For this review, take the finished solid that the model builds, in its own axes (mm). Face numbers are marked on the shaded views. A direction names the side the tool comes from. Coordinates: 2 decimals unless noted, no trailing zeros. Order: outer loops, then holes, each group sorted by start corner. A loop starts at its lowest first (then second) coordinate and runs counter-clockwise, first axis right, second up. Notation, with made-up numbers: (-39, 62.5) -> (13, 62.5) arc R11 cw to (13, 75.5) -> close; hole circle Ø10 at (70, 45.25). An arc over 180 degrees is marked (long way). Answer as a JSON object with one key per item and string values. Group by question number.
1) Draft analysis for pull direction X (two halves, no side actions). For the marked faces 1, 2, 3 and 4, state which applies: +X half, -X half, draft (parallel to the pull), parting line (faces both ways), or undercut.
2) Add section B-B, the plane y = -16. Count the separate pieces of the cut face and the enclosed holes in it, then the cut area to 3 significant figures.
3) Add section A-A, the plane z = 1.25. Write out the cut boundary in (x, y), then the cut area to 3 significant figures.
4) Machinability: for the marked faces 5 and 6, which of the approach directions +Z, -Z, +X, -X, +Y, -Y give a long, thin tool a straight path to every point of the face, cutting with its end or side? Answer none if there is none.
5) Wall thickness on L1, parallel to X at y = 12.5, z = 1; L2, parallel to Y at x = -24.5, z = 2; L3, parallel to Z at x = 32, y = -12.5: over which ranges is each line inside the solid? List them lowest first.
6) For pin 1 (6.5 mm diameter, centred on x = 0, y = 24, fed in from -Z); pin 2 (11 mm diameter, centred on x = 0, y = -8, fed in from +Z), all flat-tipped, find the tip position at first contact; note any pin that passes through.
from build123d import *

# Parameters (mm, degrees)
EXTRUDE_THIN1_DEPTH       = 10
BOSS_EXTRUDE1_DEPTH       = 2
SKETCH3_W                 = 3
SKETCH3_H                 = 56
BOSS_EXTRUDE2_DEPTH       = 6.5
SKETCH4_W                 = 9
SKETCH4_H                 = 56
BOSS_EXTRUDE3_DEPTH       = 5
F_3_0MM_DOWEL_HOLE1_D     = 3
F_3_0MM_DOWEL_HOLE1_DEPTH = 150
SKETCH10_R                = 3.5
CUT_EXTRUDE1_DEPTH        = 65.195015383
CUT_EXTRUDE1_DEPTH_BACK   = 65.195015383
BOSS_EXTRUDE4_REACH       = 105.179
SKETCH12_W                = 9
SKETCH12_H                = 56
SKETCH12_R                = 1.5
BOSS_EXTRUDE5_REACH       = 105.179
SKETCH13_W                = 9
SKETCH13_H                = 56
SKETCH13_R                = 1.5
SKETCH14_R                = 1.5
CUT_EXTRUDE2_DEPTH        = 104.179455319
CUT_EXTRUDE2_DEPTH_BACK   = 104.179455319
SKETCH15_R                = 1.5
SKETCH15_R_2              = 1.2
BOSS_EXTRUDE6_DEPTH       = 8.5
BOSS_EXTRUDE7_START       = -100
SKETCH15_2_R              = 1.5
SKETCH15_2_R_2            = 1.2
BOSS_EXTRUDE7_DEPTH       = 8.5


with BuildPart() as part:
    # Sketch1 → Extrude-Thin1 (new body)
    with BuildSketch(Plane.XY):
        with BuildLine():
            Line((-35.5, 39), (35.5, 39))
            ThreePointArc((35.5, 39), (41.156854249, 36.656854249), (43.5, 31))
            Line((43.5, 31), (43.5, -31))
            ThreePointArc((43.5, -31), (41.156854249, -36.656854249), (35.5, -39))
            Line((35.5, -39), (-35.5, -39))
            ThreePointArc((-35.5, -39), (-41.156854249, -36.656854249), (-43.5, -31))
            Line((-43.5, -31), (-43.5, 31))
            ThreePointArc((-43.5, 31), (-41.156854249, 36.656854249), (-35.5, 39))
        make_face()
        with BuildLine():
            Line((-35.5, 37), (35.5, 37))
            ThreePointArc((35.5, 37), (39.742640687, 35.242640687), (41.5, 31))
            Line((41.5, 31), (41.5, -31))
            ThreePointArc((41.5, -31), (39.742640687, -35.242640687), (35.5, -37))
            Line((35.5, -37), (-35.5, -37))
            ThreePointArc((-35.5, -37), (-39.742640687, -35.242640687), (-41.5, -31))
            Line((-41.5, -31), (-41.5, 31))
            ThreePointArc((-41.5, 31), (-39.742640687, 35.242640687), (-35.5, 37))
        make_face(mode=Mode.SUBTRACT)
    extrude(amount=EXTRUDE_THIN1_DEPTH)

    # Sketch2 → Boss-Extrude1 (add)
    with BuildSketch(Plane(origin=(0, 0, 0), x_dir=(-1, 0, 0), z_dir=(0, 0, -1))):
        with BuildLine():
            Line((35.5, 39), (-35.5, 39))
            ThreePointArc((-35.5, 39), (-41.156854249, 36.656854249), (-43.5, 31))
            Line((-43.5, 31), (-43.5, -31))
            ThreePointArc((-43.5, -31), (-41.156854249, -36.656854249), (-35.5, -39))
            Line((-35.5, -39), (35.5, -39))
            ThreePointArc((35.5, -39), (41.156854249, -36.656854249), (43.5, -31))
            Line((43.5, -31), (43.5, 31))
            ThreePointArc((43.5, 31), (41.156854249, 36.656854249), (35.5, 39))
        make_face()
        with BuildLine():
            ThreePointArc((-35.5, -37), (-39.742640687, -35.242640687), (-41.5, -31))
            Line((-41.5, -31), (-41.5, 31))
            ThreePointArc((-41.5, 31), (-39.742640687, 35.242640687), (-35.5, 37))
            Line((-35.5, 37), (35.5, 37))
            ThreePointArc((35.5, 37), (39.742640687, 35.242640687), (41.5, 31))
            Line((41.5, 31), (41.5, -31))
            ThreePointArc((41.5, -31), (39.742640687, -35.242640687), (35.5, -37))
            Line((35.5, -37), (-35.5, -37))
        make_face(mode=Mode.SUBTRACT)
        with BuildLine():
            Line((-41.5, -31), (-41.5, 31))
            ThreePointArc((-41.5, 31), (-39.742640687, 35.242640687), (-35.5, 37))
            Line((-35.5, 37), (35.5, 37))
            ThreePointArc((35.5, 37), (39.742640687, 35.242640687), (41.5, 31))
            Line((41.5, 31), (41.5, -31))
            ThreePointArc((41.5, -31), (39.742640687, -35.242640687), (35.5, -37))
            Line((35.5, -37), (-35.5, -37))
            ThreePointArc((-35.5, -37), (-39.742640687, -35.242640687), (-41.5, -31))
        make_face()
    extrude(amount=BOSS_EXTRUDE1_DEPTH)

    # Sketch3 → Boss-Extrude2 (add)
    with BuildSketch(Plane.ZY.offset(43.5)):
        with Locations((-0.5, 0)):
            Rectangle(SKETCH3_W, SKETCH3_H)
    boss_extrude2 = extrude(amount=BOSS_EXTRUDE2_DEPTH)

    # Sketch4 → Boss-Extrude3 (add)
    with BuildSketch(Plane.ZY.offset(50)):
        with Locations((5.5, 0)):
            Rectangle(SKETCH4_W, SKETCH4_H)
    boss_extrude3 = extrude(amount=-BOSS_EXTRUDE3_DEPTH)

    # Ø3.0mm Dowel Hole1
    with Locations(Plane(origin=(-50, -6.5, 5.5), x_dir=(0, 0, -1), z_dir=(-1, 0, 0))):
        with Locations((0, 0), (0, -13)):
            Hole(F_3_0MM_DOWEL_HOLE1_D / 2, depth=F_3_0MM_DOWEL_HOLE1_DEPTH)

    # Mirror2: Boss-Extrude2, Boss-Extrude3 across plane
    add(boss_extrude2.mirror(Plane(origin=(0, 0, 0), x_dir=(0, 0, 1), z_dir=(1, 0, 0))))
    add(boss_extrude3.mirror(Plane(origin=(0, 0, 0), x_dir=(0, 0, 1), z_dir=(1, 0, 0))))

    # Sketch10 → Cut-Extrude1 (cut, two sides)
    with BuildSketch(Plane.XY) as cut_extrude1_sk:
        with Locations((-27.375, 32)):
            Circle(SKETCH10_R)
        with Locations((-18.25, 32)):
            Circle(SKETCH10_R)
        with Locations((-9.125, 32)):
            Circle(SKETCH10_R)
        with Locations((0, 32)):
            Circle(SKETCH10_R)
        with Locations((-36.5, 32)):
            Circle(SKETCH10_R)
        with Locations((9.125, 32)):
            Circle(SKETCH10_R)
        with Locations((-27.375, 24)):
            Circle(SKETCH10_R)
        with Locations((-18.25, 24)):
            Circle(SKETCH10_R)
        with Locations((-9.125, 24)):
            Circle(SKETCH10_R)
        with Locations((0, 24)):
            Circle(SKETCH10_R)
        with Locations((9.125, 24)):
            Circle(SKETCH10_R)
        with Locations((-27.375, 16)):
            Circle(SKETCH10_R)
        with Locations((-18.25, 16)):
            Circle(SKETCH10_R)
        with Locations((-9.125, 16)):
            Circle(SKETCH10_R)
        with Locations((0, 16)):
            Circle(SKETCH10_R)
        with Locations((9.125, 16)):
            Circle(SKETCH10_R)
        with Locations((-27.375, 8)):
            Circle(SKETCH10_R)
        with Locations((-18.25, 8)):
            Circle(SKETCH10_R)
        with Locations((-9.125, 8)):
            Circle(SKETCH10_R)
        with Locations((0, 8)):
            Circle(SKETCH10_R)
        with Locations((9.125, 8)):
            Circle(SKETCH10_R)
        with Locations((-27.375, 0)):
            Circle(SKETCH10_R)
        with Locations((-18.25, 0)):
            Circle(SKETCH10_R)
        with Locations((-9.125, 0)):
            Circle(SKETCH10_R)
        Circle(SKETCH10_R)
        with Locations((9.125, 0)):
            Circle(SKETCH10_R)
        with Locations((-36.5, 24)):
            Circle(SKETCH10_R)
        with Locations((-36.5, 16)):
            Circle(SKETCH10_R)
        with Locations((-36.5, 8)):
            Circle(SKETCH10_R)
        with Locations((-36.5, 0)):
            Circle(SKETCH10_R)
        with Locations((-36.5, -8)):
            Circle(SKETCH10_R)
        with Locations((-27.375, -8)):
            Circle(SKETCH10_R)
        with Locations((-18.25, -8)):
            Circle(SKETCH10_R)
        with Locations((-9.125, -8)):
            Circle(SKETCH10_R)
        with Locations((0, -8)):
            Circle(SKETCH10_R)
        with Locations((9.125, -8)):
            Circle(SKETCH10_R)
        with Locations((-36.5, -16)):
            Circle(SKETCH10_R)
        with Locations((-27.375, -16)):
            Circle(SKETCH10_R)
        with Locations((-18.25, -16)):
            Circle(SKETCH10_R)
        with Locations((-9.125, -16)):
            Circle(SKETCH10_R)
        with Locations((0, -16)):
            Circle(SKETCH10_R)
        with Locations((9.125, -16)):
            Circle(SKETCH10_R)
        with Locations((-36.5, -24)):
            Circle(SKETCH10_R)
        with Locations((-27.375, -24)):
            Circle(SKETCH10_R)
        with Locations((-18.25, -24)):
            Circle(SKETCH10_R)
        with Locations((-9.125, -24)):
            Circle(SKETCH10_R)
        with Locations((0, -24)):
            Circle(SKETCH10_R)
        with Locations((9.125, -24)):
            Circle(SKETCH10_R)
        with Locations((-36.5, -32)):
            Circle(SKETCH10_R)
        with Locations((-27.375, -32)):
            Circle(SKETCH10_R)
        with Locations((-18.25, -32)):
            Circle(SKETCH10_R)
        with Locations((-9.125, -32)):
            Circle(SKETCH10_R)
        with Locations((0, -32)):
            Circle(SKETCH10_R)
        with Locations((9.125, -32)):
            Circle(SKETCH10_R)
        with Locations((18.25, 32)):
            Circle(SKETCH10_R)
        with Locations((27.375, 32)):
            Circle(SKETCH10_R)
        with Locations((36.5, 32)):
            Circle(SKETCH10_R)
        with Locations((18.25, 24)):
            Circle(SKETCH10_R)
        with Locations((27.375, 24)):
            Circle(SKETCH10_R)
        with Locations((36.5, 24)):
            Circle(SKETCH10_R)
        with Locations((18.25, 16)):
            Circle(SKETCH10_R)
        with Locations((27.375, 16)):
            Circle(SKETCH10_R)
        with Locations((36.5, 16)):
            Circle(SKETCH10_R)
        with Locations((18.25, 8)):
            Circle(SKETCH10_R)
        with Locations((27.375, 8)):
            Circle(SKETCH10_R)
        with Locations((36.5, 8)):
            Circle(SKETCH10_R)
        with Locations((18.25, 0)):
            Circle(SKETCH10_R)
        with Locations((27.375, 0)):
            Circle(SKETCH10_R)
        with Locations((36.5, 0)):
            Circle(SKETCH10_R)
        with Locations((18.25, -8)):
            Circle(SKETCH10_R)
        with Locations((27.375, -8)):
            Circle(SKETCH10_R)
        with Locations((36.5, -8)):
            Circle(SKETCH10_R)
        with Locations((18.25, -16)):
            Circle(SKETCH10_R)
        with Locations((27.375, -16)):
            Circle(SKETCH10_R)
        with Locations((36.5, -16)):
            Circle(SKETCH10_R)
        with Locations((18.25, -24)):
            Circle(SKETCH10_R)
        with Locations((27.375, -24)):
            Circle(SKETCH10_R)
        with Locations((36.5, -24)):
            Circle(SKETCH10_R)
        with Locations((18.25, -32)):
            Circle(SKETCH10_R)
        with Locations((27.375, -32)):
            Circle(SKETCH10_R)
        with Locations((36.5, -32)):
            Circle(SKETCH10_R)
    extrude(amount=CUT_EXTRUDE1_DEPTH, mode=Mode.SUBTRACT)
    extrude(cut_extrude1_sk.sketch, amount=-CUT_EXTRUDE1_DEPTH_BACK, mode=Mode.SUBTRACT)

    # Sketch12 → Boss-Extrude4 (add, up to next)
    with BuildSketch(Plane(origin=(-45, 0, 0), x_dir=(0, 0, -1), z_dir=(1, 0, 0)), mode=Mode.PRIVATE) as boss_extrude4_sk1:
        with Locations((-5.5, 0)):
            Rectangle(SKETCH12_W, SKETCH12_H)
        with Locations(Location((-5.5, 6.5, 0), (0, 0, 180))):
            Circle(SKETCH12_R, mode=Mode.SUBTRACT)
        with Locations(Location((-5.5, -6.5, 0), (0, 0, 180))):
            Circle(SKETCH12_R, mode=Mode.SUBTRACT)
    boss_extrude4_tool1 = extrude(boss_extrude4_sk1.sketch, amount=BOSS_EXTRUDE4_REACH, mode=Mode.PRIVATE) - part.part
    add(boss_extrude4_tool1.solids().sort_by_distance((-45, 0, 5.5))[0])

    # Sketch13 → Boss-Extrude5 (add, up to next)
    with BuildSketch(Plane.ZY.offset(-45), mode=Mode.PRIVATE) as boss_extrude5_sk1:
        with Locations((5.5, 0)):
            Rectangle(SKETCH13_W, SKETCH13_H)
        with Locations((5.5, 6.5)):
            Circle(SKETCH13_R, mode=Mode.SUBTRACT)
        with Locations((5.5, -6.5)):
            Circle(SKETCH13_R, mode=Mode.SUBTRACT)
    boss_extrude5_tool1 = extrude(boss_extrude5_sk1.sketch, amount=BOSS_EXTRUDE5_REACH, mode=Mode.PRIVATE) - part.part
    add(boss_extrude5_tool1.solids().sort_by_distance((45, 0, 5.5))[0])

    # Sketch14 → Cut-Extrude2 (cut, two sides)
    with BuildSketch(Plane.ZY.offset(-45)) as cut_extrude2_sk:
        with Locations((5.5, -6.5)):
            Circle(SKETCH14_R)
        with Locations((5.5, 6.5)):
            Circle(SKETCH14_R)
    extrude(amount=CUT_EXTRUDE2_DEPTH, mode=Mode.SUBTRACT)
    extrude(cut_extrude2_sk.sketch, amount=-CUT_EXTRUDE2_DEPTH_BACK, mode=Mode.SUBTRACT)

    # Sketch15 → Boss-Extrude6 (add)
    with BuildSketch(Plane.ZY.offset(50)):
        with Locations((5.5, 6.5)):
            Circle(SKETCH15_R)
        with Locations((5.5, 6.5)):
            Circle(SKETCH15_R_2, mode=Mode.SUBTRACT)
        with Locations((5.5, -6.5)):
            Circle(SKETCH15_R)
        with Locations((5.5, -6.5)):
            Circle(SKETCH15_R_2, mode=Mode.SUBTRACT)
    extrude(amount=-BOSS_EXTRUDE6_DEPTH)

    # Sketch15<2> → Boss-Extrude7 (add)
    with BuildSketch(Plane.ZY.offset(50).offset(BOSS_EXTRUDE7_START)):
        with Locations((5.5, 6.5)):
            Circle(SKETCH15_2_R)
        with Locations((5.5, 6.5)):
            Circle(SKETCH15_2_R_2, mode=Mode.SUBTRACT)
        with Locations((5.5, -6.5)):
            Circle(SKETCH15_2_R)
        with Locations((5.5, -6.5)):
            Circle(SKETCH15_2_R_2, mode=Mode.SUBTRACT)
    extrude(amount=BOSS_EXTRUDE7_DEPTH)


solid = part.part
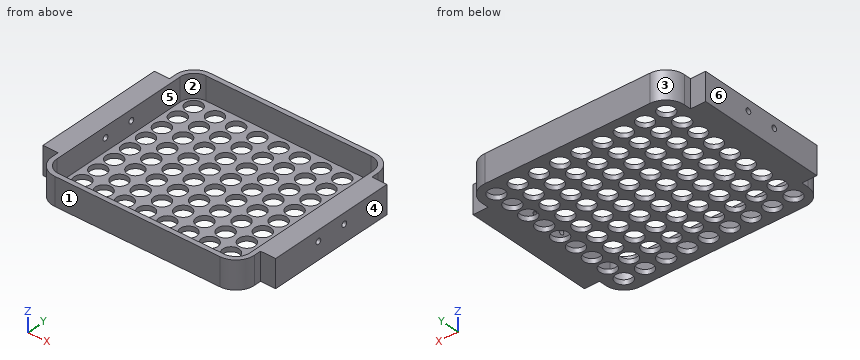
Output values:
{
 "1": {"face 1": "draft", "face 2": "undercut", "face 3": "-X half", "face 4": "+X half"},
 "2": {"separate pieces": "10", "enclosed holes": "0", "area": "244 mm²"},
 "3": {"outline": "(-50, -28) -> (-43.5, -28) -> (-43.5, -31) arc R8 ccw to (-35.5, -39) -> (35.5, -39) arc R8 ccw to (43.5, -31) -> (43.5, -28) -> (50, -28) -> (50, 28) -> (43.5, 28) -> (43.5, 31) arc R8 ccw to (35.5, 39) -> (-35.5, 39) arc R8 ccw to (-43.5, 31) -> (-43.5, 28) -> (-50, 28) -> close; hole (-41.5, -31) arc R6 ccw to (-35.5, -37) -> (35.5, -37) arc R6 ccw to (41.5, -31) -> (41.5, 31) arc R6 ccw to (35.5, 37) -> (-35.5, 37) arc R6 ccw to (-41.5, 31) -> close", "area": "1,350 mm²"},
 "4": {"face 5": "+Z", "face 6": "+Z, -Z, -X, +Y, -Y"},
 "5": {"L1": "x = -50 to -41.5, 41.5 to 50", "L2": "y = -39 to -37, 37 to 39", "L3": "z = -2 to 0"},
 "6": {"pin 1": "passes through", "pin 2": "stops at z = 0"}
}
